CAD build for the part. Positions are in the model's coordinates, mm. A direction names the side the tool comes from. Round coordinates to 2 decimals unless told otherwise and drop trailing zeros. Order: outer loops, then holes, each group sorted by start corner. A loop starts at its lowest first (then second) coordinate and runs counter-clockwise, first axis right, second up. Notation, with made-up numbers: (76.25, -40) - (112.25, -40) arc R20 ccw to (112.25, -28) - close; hole circle Ø5 at (52, -2). An arc over 180 degrees is marked (long way). Write item = value, one per line.
from build123d import *

# Parameters (mm, degrees)
BOSS_EXTRU_1_DEPTH           = 10
ESQUISSE2_W                  = 10.2
ESQUISSE2_H                  = 6
ENL_V_MAT_EXTRU_1_DEPTH      = 20
CHANFREIN1_SIZE              = 2.5
CHANFREIN2_SIZE              = 1.8
CHANFREIN1_OF_SYM_TRIE1_SIZE = 2.5
CHANFREIN2_OF_SYM_TRIE1_SIZE = 1.8
ESQUISSE3_R                  = 6.5
ENL_V_MAT_EXTRU_2_DEPTH      = 32.368774283
ESQUISSE4_R                  = 7.5
ENL_V_MAT_EXTRU_3_DEPTH      = 7
CHANFREIN3_SIZE              = 1
ESQUISSE5_R                  = 1.6
ENL_V_MAT_EXTRU_4_DEPTH      = 7
CHANFREIN4_SIZE              = 2.1
CHANFREIN5_SIZE              = 2


with BuildPart() as part:
    # Esquisse1 → Boss.-Extru.1 (new body)
    with BuildSketch(Plane(origin=(0, 0, 0), x_dir=(1, 0, 0), z_dir=(0, 1, 0))):
        with BuildLine():
            Line((7.141428429, 7), (28, 7))
            Line((28, 7), (28, -7))
            Line((28, -7), (7.141428429, -7))
            ThreePointArc((7.141428429, -7), (0, -10), (-7.141428429, -7))
            Line((-7.141428429, -7), (-28, -7))
            Line((-28, -7), (-28, 7))
            Line((-28, 7), (-7.141428429, 7))
            ThreePointArc((-7.141428429, 7), (0, 10), (7.141428429, 7))
        make_face()
    extrude(amount=BOSS_EXTRU_1_DEPTH)

    # Esquisse2 → Enlèv. mat.-Extru.1 (cut)
    with BuildSketch(Plane.ZY.offset(28)):
        with Locations((0, 7)):
            Rectangle(ESQUISSE2_W, ESQUISSE2_H)
    enl_v_mat_extru_1 = extrude(amount=-ENL_V_MAT_EXTRU_1_DEPTH, mode=Mode.SUBTRACT)

    # Chanfrein1
    chanfrein1_edges = [part.edges().sort_by_distance(p)[0] for p in [
        (-18, 4, -5.1),
        (-18, 4, 5.1),
    ]]
    chamfer(chanfrein1_edges, length=CHANFREIN1_SIZE)

    # Chanfrein2
    chanfrein2_edges = [part.edges().sort_by_distance(p)[0] for p in [
        (-8, 4, 0),
        (-8, 5.25, -3.85),
        (-8, 5.25, 3.85),
    ]]
    chamfer(chanfrein2_edges, length=CHANFREIN2_SIZE)

    # Symétrie1: Enlèv. mat.-Extru.1 across plane
    add(enl_v_mat_extru_1.mirror(Plane(origin=(0, 0, 0), x_dir=(0, 0, 1), z_dir=(1, 0, 0))), mode=Mode.SUBTRACT)

    # Chanfrein1 of Symétrie1
    chanfrein1_of_sym_trie1_edges = [part.edges().sort_by_distance(p)[0] for p in [
        (18, 4, -5.1),
        (18, 4, 5.1),
    ]]
    chamfer(chanfrein1_of_sym_trie1_edges, length=CHANFREIN1_OF_SYM_TRIE1_SIZE)

    # Chanfrein2 of Symétrie1
    chanfrein2_of_sym_trie1_edges = [part.edges().sort_by_distance(p)[0] for p in [
        (8, 4, 0),
        (8, 5.25, -3.85),
        (8, 5.25, 3.85),
    ]]
    chamfer(chanfrein2_of_sym_trie1_edges, length=CHANFREIN2_OF_SYM_TRIE1_SIZE)

    # Esquisse3 → Enlèv. mat.-Extru.2 (cut, through all)
    with BuildSketch(Plane.XZ):
        with Locations(Location((0, 0, 0), (0, 0, 270))):
            Circle(ESQUISSE3_R)
    extrude(amount=-ENL_V_MAT_EXTRU_2_DEPTH, mode=Mode.SUBTRACT)

    # Esquisse4 → Enlèv. mat.-Extru.3 (cut)
    with BuildSketch(Plane.XZ):
        with Locations(Location((0, 0, 0), (0, 0, 270))):
            Circle(ESQUISSE4_R)
    extrude(amount=-ENL_V_MAT_EXTRU_3_DEPTH, mode=Mode.SUBTRACT)

    # Chanfrein3
    chanfrein3_edges = [part.edges().sort_by_distance(p)[0] for p in [
        (0, 0, 7.5),
    ]]
    chamfer(chanfrein3_edges, length=CHANFREIN3_SIZE)

    # Esquisse5 → Enlèv. mat.-Extru.4 (cut)
    with BuildSketch(Plane.XZ):
        with Locations(Location((-23, 0, 0), (0, 0, 270))):
            Circle(ESQUISSE5_R)
        with Locations(Location((-13, 0, 0), (0, 0, 270))):
            Circle(ESQUISSE5_R)
        with Locations(Location((13, 0, 0), (0, 0, 270))):
            Circle(ESQUISSE5_R)
        with Locations(Location((23, 0, 0), (0, 0, 270))):
            Circle(ESQUISSE5_R)
    extrude(amount=-ENL_V_MAT_EXTRU_4_DEPTH, mode=Mode.SUBTRACT)

    # Chanfrein4
    chanfrein4_edges = [part.edges().sort_by_distance(p)[0] for p in [
        (-23, 0, 1.6),
        (-13, 0, 1.6),
        (13, 0, 1.6),
        (23, 0, 1.6),
    ]]
    chamfer(chanfrein4_edges, length=CHANFREIN4_SIZE)

    # Chanfrein5
    chanfrein5_edges = [part.edges().sort_by_distance(p)[0] for p in [
        (28, 5, -7),
        (28, 5, 7),
        (-28, 5, -7),
        (-28, 5, 7),
    ]]
    chamfer(chanfrein5_edges, length=CHANFREIN5_SIZE)


solid = part.part
(1) Band-saw the part on B-B on y = 4.5. List the corners of the cut face in (x, z).
Solved:
outline = (-28, -5) - (-26, -7) - (-7.14, -7) arc R10 ccw to (7.14, -7) - (26, -7) - (28, -5) - (28, -3.1) - (9.8, -3.1) - (9.3, -2.39) - (9.3, 2.39) - (9.8, 3.1) - (28, 3.1) - (28, 5) - (26, 7) - (7.14, 7) arc R10 ccw to (-7.14, 7) - (-26, 7) - (-28, 5) - (-28, 3.1) - (-9.8, 3.1) - (-9.3, 2.39) - (-9.3, -2.39) - (-9.8, -3.1) - (-28, -3.1) - close; hole circle Ø15 at (0, 0)
(2) Tool access for faces 4 (the flat face through (8, 8, 0)), 5 (the flat face through (28, 2, 0)), 6 (the flat face through (17, 5, 7)), 7 (the flat face through (-19, 5.2, -3.8)), 8 (the cylindrical face through (0, 5, -10)): list every direction of +Z, -Z, +X, -X, +Y, -Y with a clear straight run to the whole face (end or side of a thin tool).
Solved:
face_4 = +X, +Y
face_5 = +Z, -Z, +X, +Y, -Y
face_6 = +Z, +X, +Y, -Y
face_7 = -X, +Y
face_8 = -Z, +Y, -Y
(3) Probe line 1 along X through (y, z) = (3.05, 0); line 2 along X through (y, z) = (4.5, 0); line 3 along X through (y, z) = (6.25, -2.25). List the from-to ranges inside material, lowest first.
Solved:
line_1 = -28 to -24.6, -21.4 to -14.6, -11.4 to -7.5, 7.5 to 11.4, 14.6 to 21.4, 24.6 to 28
line_2 = -9.3 to -7.5, 7.5 to 9.3
line_3 = -8 to -7.15, 7.15 to 8
(4) Band-saw the part on A-A on x = 13. List the corners of the cut face in (y, z), plus the area to 3 significant figures.
Solved:
outline = (0, -7) - (10, -7) - (10, -5.1) - (6.5, -5.1) - (4, -2.6) - (4, -1.6) - (2.1, -1.6) - (0, -3.7) - close; (0, 3.7) - (2.1, 1.6) - (4, 1.6) - (4, 2.6) - (6.5, 5.1) - (10, 5.1) - (10, 7) - (0, 7) - close
area = 67.8 mm²
(5) Band-saw the part on C-C on z = 0. Count the separate pieces of the cut face and the enclosed holes in it, plus the area to 3 significant figures.
Solved:
separate_pieces = 6
enclosed_holes = 0
area = 109 mm²
(6) Band-saw the part on D-D on x = -17.5. List the corners of the cut face in (y, z), plus the area to 4 significant figures.
Solved:
outline = (0, -7) - (10, -7) - (10, -5.1) - (6.5, -5.1) - (4, -2.6) - (4, 2.6) - (6.5, 5.1) - (10, 5.1) - (10, 7) - (0, 7) - close
area = 85.05 mm²
(7) Pull direction X, two halves, no side cores. Call faces 1 (the cylindrical face through (14.586, 3.037, 0.208)), 2 (the flat face through (6.3, 10, -2.3)), 3 (the flat face through (8.89, 6.14, -3.45)): released by +X, released by -X, zero draft, split by the parting line, or undercut.
Solved:
face_1 = undercut
face_2 = zero draft
face_3 = released by +X
(8) Drop flat-ended pins along their axis: pin 1 (3.5 mm diameter, centred on y = 8.5, z = 2, fed in from +X); pin 2 (4 mm diameter, centred on x = 13, z = 0, fed in from +Y); pin 3 (3 mm diameter, centred on x = -20, y = 8, fed in from -Z); pin 4 (7.5 mm diameter, centred on x = -0.5, z = -2, fed in from -Y). Give the stop position or say it passes through.
Solved:
pin_1 = 8
pin_2 = 4
pin_3 = -7
pin_4 = through
